Source: CAD feature listing. Evaluate the final solid. Frame: model axes, mm. A direction names the side the tool comes from. Give positions to 0.01 mm unless a question says otherwise; leave off trailing zeros. Loops run counter-clockwise (first coordinate to the right, second up) from the corner with the lowest first, then second, coordinate; pieces in that order, holes last. Notation, with made-up numbers: M 26,-35.5 L 40,-35.5 A12 ccw 40,-18.5 Z; hole C 37,-26 d4. An arc over 180 degrees is marked long. Put each result on its own line as item: value.
from build123d import *

# Parameters (mm, degrees)
F1_DEPTH = 25
F2_W     = 4
F2_H     = 71.1512080157
F3_DEPTH = 25
F4_R     = 3
F5_DEPTH = 25


with BuildPart() as f1:
    # F0 (on Front) → F1 (new body)
    with BuildSketch(Plane.XZ):
        Polygon((9, -73.9955009194), (12, -73.9955009194), (12, -2.8442929037), (3.6967449024, 6.3815460937), (3.6967449024, 9.0044990806), (-3.6967449024, 9.0044990806), (-3.6967449024, 6.3815460937), (-12, -2.8442929037), (-12, -73.9955009194), (-9, -73.9955009194), (-9, -3.9955009194), (0, 6.0044990806), (9, -3.9955009194), align=None)
    extrude(amount=F1_DEPTH)

    # F2 (on face) → F3 (cut)
    with BuildSketch(Plane.YZ.offset(12)):
        with Locations((-23, -38.4198969115)):
            Rectangle(F2_W, F2_H)
        with Locations((-2, -38.4198969115)):
            Rectangle(F2_W, F2_H)
        Polygon((-4, 9.0044990806), (-4, -2.8442929037), (0, -2.8442929037), (0, -73.9955009194), (3.3893596847, -73.9955009194), (3.3893596847, 9.0044990806), align=None)
        Polygon((-25, -2.8442929037), (-21, -2.8442929037), (-21, 9.0044990806), (-27.9794055969, 9.0044990806), (-27.9794055969, -73.9955009194), (-25, -73.9955009194), align=None)
    extrude(amount=-F3_DEPTH, mode=Mode.SUBTRACT)

    # F4 (on face) → F5 (cut)
    with BuildSketch(Plane.YZ.offset(12)):
        with BuildLine():
            ThreePointArc((-12.5, -73.9955009194), (-18.5104076401, -71.5059085594), (-21, -65.4955009194))
            Line((-21, -65.4955009194), (-21, -73.9955009194))
            Line((-21, -73.9955009194), (-12.5, -73.9955009194))
        make_face()
        with BuildLine():
            ThreePointArc((-4, -65.4955009194), (-6.4895923599, -71.5059085594), (-12.5, -73.9955009194))
            Line((-12.5, -73.9955009194), (-4, -73.9955009194))
            Line((-4, -73.9955009194), (-4, -65.4955009194))
        make_face()
        with Locations((-12.5, -65.4955009194)):
            Circle(F4_R)
        with Locations((-12.5, -13.4955009194)):
            Circle(F4_R)
    extrude(amount=-F5_DEPTH, mode=Mode.SUBTRACT)


solid = f1.part
1. Section query D-D (z = 3.5). Output: boundary loops of the cut face in (x, y), plus the area to 3 significant figures.
Found:
outline: M -6.29,-21 L -2.25,-21 L -2.25,-4 L -6.29,-4 Z; M 2.25,-21 L 6.29,-21 L 6.29,-4 L 2.25,-4 Z
area: 137 mm^2
2. Section query C-C (y = -11.5). State how many separate pieces and enclosed holes the cut face has, plus the area to 3 significant figures.
Found:
separate pieces: 5
enclosed holes: 0
area: 454 mm^2
3. Section query B-B (x = -10.5). Output: boundary loops of the cut face in (y, z).
Found:
outline: M -21,-65.5 A8.5 ccw -4,-65.5 L -4,-1.18 L -21,-1.18 Z; hole C -12.5,-65.5 d6; hole C -12.5,-13.5 d6
4. Access query for faces 5 (the cylindrical face through (10.52, -14.88, -67.32)), 6 (the flat face through (4.44, -12.38, 1.07)), 7 (the flat face through (3.697, -12, 8)), 8 (the flat face through (-3.697, -12, 8)). Directions: +Z, -Z, +X, -X, +Y, -Y. A direction counts if a zero-diameter tool reaches every point of the face in a straight line with its end or side. Return the directions, or none.
Found:
face 5: +X, -X
face 6: -Z, +Y, -Y
face 7: +Z, +X, +Y, -Y
face 8: +Z, -X, +Y, -Y
5. Contact query for flat-ended pins moving along their axis: P1, Ø1.3, axis at y = -12, z = 7, coming from the +X side; P2, Ø1.3, axis at y = -16.5, z = 7, coming from the -X side. Output: stop coordinate, or through.
Found:
P1: x = 3.73
P2: x = -3.73
6. Section query A-A (z = -33). Output: boundary loops of the cut face in (x, y).
Found:
outline: M -12,-21 L -9,-21 L -9,-4 L -12,-4 Z; M 9,-21 L 12,-21 L 12,-4 L 9,-4 Z
7. Material intervals for line 1 (X direction, y = -7.25, z = -53); line 2 (Z direction, x = 10.25, y = -13.75); line 3 (Z direction, x = 10.95, y = -12.5), sorted ascending. Write a range as from..to.
Found:
line 1: -12..-9, 9..12
line 2: -73.9..-68.22, -62.77..-16.22, -10.77..-0.9
line 3: -74..-68.5, -62.5..-16.5, -10.5..-1.68
8. Draft query along Y for faces 1 (the cylindrical face through (10.52, -14.88, -15.32)), 2 (the flat face through (-4.563, -12.381, 0.934)), 3 (the flat face through (10, -21, -26)), 4 (the flat face through (10, -4, -25)). Return one class per face: pulls with the +Y half, pulls with the -Y half, needs draft (parallel to the pull), parting line crosses it, or undercut.
Found:
face 1: undercut
face 2: needs draft
face 3: pulls with the -Y half
face 4: pulls with the +Y half
